Geometry: final body of the model. Coordinates: model frame, mm. A direction names the side the tool comes from. Round coordinates to 2 decimals unless told otherwise and drop trailing zeros. Loops run counter-clockwise (first coordinate to the right, second up) from the corner with the lowest first, then second, coordinate; pieces in that order, holes last. Notation, with made-up numbers: (75, 80) - (83, 80) arc R20 ccw to (83, 94) - close; hole circle Ø8 at (74, 83.25). An arc over 180 degrees is marked (long way). Answer as a JSON object with one key per item and string values. Group by question number.
Item 1: Draft query along X for faces 3 (the face through (32.466, 48.487, -12.836)), 4 (the face through (9.273, 4.93, -17.314)), 5 (the face through (13.25, 48, -13)). Return one class per face: released by +X, released by -X, zero draft, split by the parting line, or undercut.
Item 2: Section C-C (y = 80). Return the cut outline in (x, z), plus the area to 3 significant figures.
Item 3: Section D-D (x = 27). Return the cut outline in (y, z), plus the area to 3 significant figures.
Item 4: Section A-A (y = 67). Return the cut outline in (x, z), plus the area to 4 significant figures.
Item 5: First-contact query: pin 1 (3 mm diameter, centred on y = 70, z = -12.5, fed in from +X); pin 2 (6 mm diameter, centred on x = 5.5, z = -7.5, fed in from +Y); pin 3 (3 mm diameter, centred on y = 27.5, z = -15.5, fed in from -X). Flat tips, straight axial feed; report the tip coordinate or a pass-through.
Item 6: Line query: line 1 (X direction, y = 71, z = -9.5); line 2 (Z direction, x = 19.25, y = 60); line 3 (X direction, y = 15.5, z = -18.5). Output: solid intervals per line, ascending.
Item 7: Reachability of faces 1 (the face through (0, 5, -12)), 2 (the face through (25, 18, -12)) from +Z, -Z, +X, -X, +Y, -Y: full face, straight path, thin tool, end or side. Return the list, or none.
Item 8: Section B-B (z = -7). Return the cut outline in (x, y), plus the area to 3 significant figures.
```python
from build123d import *

# Parameters (mm, degrees)
SKETCH1_W               = 50
SKETCH1_H               = 25
BOSS_EXTRUDE1_DEPTH     = 10
SKETCH2_W               = 20
SKETCH2_H               = 25
BOSS_EXTRUDE2_DEPTH     = 75
SKETCH3_W               = 6.6
SKETCH3_H               = 25
CUT_EXTRUDE1_DEPTH      = 75
SKETCH4_R               = 1.55
CUT_EXTRUDE2_DEPTH      = 96.262794416
LPATTERN1_COUNT         = 6
LPATTERN1_PITCH         = 10
SKETCH5_W               = 15
SKETCH5_H               = 25
CUT_EXTRUDE3_DEPTH      = 94.541434669
SKETCH6_R               = 1.9
CUT_EXTRUDE4_DEPTH      = 96.262794416
SKETCH7_R               = 1.9
CUT_EXTRUDE5_DEPTH      = 87.458082329
SKETCH8_W               = 6.6
SKETCH8_H               = 8
BOSS_EXTRUDE4_DEPTH     = 25
SKETCH11_W              = 25
SKETCH11_H              = 85
BOSS_EXTRUDE5_DEPTH     = 1.75
SKETCH12_W              = 25
SKETCH12_H              = 75
BOSS_EXTRUDE6_DEPTH     = 1.75
SKETCH14_R              = 1.9
CUT_EXTRUDE7_DEPTH      = 88.18120497
CUT_EXTRUDE8_DEPTH      = 94.010160735
CUT_EXTRUDE8_DEPTH_BACK = 94.010160735
SKETCH15_R              = 1.55
CHAMFER1_SIZE           = 1


with BuildPart() as part:
    # Sketch1 → Boss-Extrude1 (new body)
    with BuildSketch(Plane(origin=(0, 0, 0), x_dir=(1, 0, 0), z_dir=(0, 1, 0))):
        with Locations((25, 12.5)):
            Rectangle(SKETCH1_W, SKETCH1_H)
    extrude(amount=BOSS_EXTRUDE1_DEPTH)

    # Sketch2 → Boss-Extrude2 (add)
    with BuildSketch(Plane(origin=(0, 10, 0), x_dir=(1, 0, 0), z_dir=(0, 1, 0))):
        with Locations((25, 12.5)):
            Rectangle(SKETCH2_W, SKETCH2_H)
    extrude(amount=BOSS_EXTRUDE2_DEPTH)

    # Sketch3 → Cut-Extrude1 (cut)
    with BuildSketch(Plane(origin=(0, 85, 0), x_dir=(1, 0, 0), z_dir=(0, 1, 0))):
        with Locations((25, 12.5)):
            Rectangle(SKETCH3_W, SKETCH3_H)
    extrude(amount=-CUT_EXTRUDE1_DEPTH, mode=Mode.SUBTRACT)

    # Sketch4 → Cut-Extrude2 (cut, symmetric)
    with BuildSketch(Plane.ZY.offset(-15)):
        with Locations((-12.5, 80)):
            Circle(SKETCH4_R)
    cut_extrude2 = extrude(amount=CUT_EXTRUDE2_DEPTH, both=True, mode=Mode.SUBTRACT)

    # LPattern1: Cut-Extrude2 ×6
    with Locations(*[(0, -i * LPATTERN1_PITCH, 0) for i in range(1, LPATTERN1_COUNT)]):
        add(cut_extrude2, mode=Mode.SUBTRACT)

    # Sketch5 → Cut-Extrude3 (cut, through all)
    with BuildSketch(Plane(origin=(0, 10, 0), x_dir=(1, 0, 0), z_dir=(0, 1, 0))):
        with Locations((42.5, 12.5)):
            Rectangle(SKETCH5_W, SKETCH5_H)
    extrude(amount=-CUT_EXTRUDE3_DEPTH, mode=Mode.SUBTRACT)

    # Sketch6 → Cut-Extrude4 (cut, through all)
    with BuildSketch(Plane.XZ):
        with Locations(Location((10.000440006, -5.930630913, 0), (0, 0, 270))):
            Circle(SKETCH6_R)
    cut_extrude4 = extrude(amount=-CUT_EXTRUDE4_DEPTH, mode=Mode.SUBTRACT)

    # Mirror1: Cut-Extrude4 across plane
    add(cut_extrude4.mirror(Plane.XY.offset(-12.5)), mode=Mode.SUBTRACT)

    # Sketch7 → Cut-Extrude5 (cut, through all)
    with BuildSketch(Plane(origin=(0, 10, 0), x_dir=(1, 0, 0), z_dir=(0, 1, 0))):
        with Locations(Location((10.000440006, 14.590630913, 0), (0, 0, 270))):
            Circle(SKETCH7_R)
        with Locations(Location((10.000440006, 5.930630913, 0), (0, 0, 90))):
            Circle(SKETCH7_R)
    extrude(amount=-CUT_EXTRUDE5_DEPTH, mode=Mode.SUBTRACT)

    # Sketch8 → Boss-Extrude4 (add, through all)
    with BuildSketch(Plane.XY):
        with Locations((25, 14)):
            Rectangle(SKETCH8_W, SKETCH8_H)
    extrude(amount=-BOSS_EXTRUDE4_DEPTH)

    # Sketch11 → Boss-Extrude5 (add)
    with BuildSketch(Plane(origin=(35, 0, 0), x_dir=(0, 0, -1), z_dir=(1, 0, 0))):
        with Locations((12.5, 42.5)):
            Rectangle(SKETCH11_W, SKETCH11_H)
    extrude(amount=BOSS_EXTRUDE5_DEPTH)

    # Sketch12 → Boss-Extrude6 (add)
    with BuildSketch(Plane.ZY.offset(-15)):
        with Locations((-12.5, 47.5)):
            Rectangle(SKETCH12_W, SKETCH12_H)
    extrude(amount=BOSS_EXTRUDE6_DEPTH)

    # Sketch14 → Cut-Extrude7 (cut, through all)
    with BuildSketch(Plane(origin=(0, 10, 0), x_dir=(1, 0, 0), z_dir=(0, 1, 0))):
        with Locations(Location((10.000440006, 10.260630913, 0), (0, 0, 270))):
            Circle(SKETCH14_R)
    extrude(amount=-CUT_EXTRUDE7_DEPTH, mode=Mode.SUBTRACT)

    # Sketch15 → Cut-Extrude8 (cut, two sides: drawn at the far end of the back side and taken through both)
    with BuildSketch(Plane.ZY.offset(-28.3).offset(-CUT_EXTRUDE8_DEPTH_BACK)):
        with Locations((-12.5, 30)):
            Circle(SKETCH15_R)
        with Locations((-12.5, 40)):
            Circle(SKETCH15_R)
        with Locations((-12.5, 50)):
            Circle(SKETCH15_R)
        with Locations((-12.5, 60)):
            Circle(SKETCH15_R)
        with Locations((-12.5, 70)):
            Circle(SKETCH15_R)
        with Locations((-12.5, 80)):
            Circle(SKETCH15_R)
    extrude(amount=CUT_EXTRUDE8_DEPTH + CUT_EXTRUDE8_DEPTH_BACK, mode=Mode.SUBTRACT)

    # Chamfer1
    chamfer1_edges = [part.edges().sort_by_distance(p)[0] for p in [
        (21.7, 51.5, -25),
        (21.7, 51.5, 0),
        (28.3, 51.5, 0),
        (28.3, 51.5, -25),
        (25, 18, -25),
        (25, 18, 0),
        (36.75, 85, -12.5),
        (36.75, 42.5, 0),
        (36.75, 0, -12.5),
        (36.75, 42.5, -25),
        (6.625, 10, -25),
        (13.25, 47.5, -25),
        (13.25, 47.5, 0),
        (13.25, 85, -12.5),
        (17.475, 85, 0),
        (32.525, 85, -25),
        (32.525, 85, 0),
        (17.475, 85, -25),
        (0, 10, -12.5),
        (18.375, 0, 0),
        (0, 0, -12.5),
        (0, 5, -25),
        (18.375, 0, -25),
        (0, 5, 0),
        (6.625, 10, 0),
    ]]
    chamfer(chamfer1_edges, length=CHAMFER1_SIZE)


solid = part.part
```
Values:
{
 "1": {"face 3": "zero draft", "face 4": "undercut", "face 5": "released by -X"},
 "2": {"outline": "(13.25, -24) - (14.25, -25) - (20.7, -25) - (21.7, -24) - (21.7, -14.05) - (13.25, -14.05) - close; (13.25, -10.95) - (21.7, -10.95) - (21.7, -1) - (20.7, 0) - (14.25, 0) - (13.25, -1) - close; (28.3, -24) - (29.3, -25) - (35.75, -25) - (36.75, -24) - (36.75, -14.05) - (28.3, -14.05) - close; (28.3, -10.95) - (36.75, -10.95) - (36.75, -1) - (35.75, 0) - (29.3, 0) - (28.3, -1) - close", "area": "366 mm^2"},
 "3": {"outline": "(0, -24) - (1, -25) - (17, -25) - (18, -24) - (18, -1) - (17, 0) - (1, 0) - (0, -1) - close", "area": "448 mm^2"},
 "4": {"outline": "(13.25, -24) - (14.25, -25) - (20.7, -25) - (21.7, -24) - (21.7, -1) - (20.7, 0) - (14.25, 0) - (13.25, -1) - close; (28.3, -24) - (29.3, -25) - (35.75, -25) - (36.75, -24) - (36.75, -1) - (35.75, 0) - (29.3, 0) - (28.3, -1) - close", "area": "418.5 mm^2"},
 "5": {"pin 1": "passes through", "pin 2": "stops at y = 10", "pin 3": "stops at x = 13.25"},
 "6": {"line 1": "x = 13.25 to 21.7, 28.3 to 36.75", "line 2": "z = -25 to -14.05, -10.95 to 0", "line 3": "x = 13.25 to 36.75"},
 "7": {"face 1": "+Z, -Z, -X, +Y, -Y", "face 2": "+Z, -Z, +Y"},
 "8": {"outline": "(0, 1) - (1, 0) - (8.43, 0) - (8.43, 10) - (1, 10) - (0, 9) - close; (11.57, 0) - (35.75, 0) - (36.75, 1) - (36.75, 84) - (35.75, 85) - (28.3, 85) - (28.3, 18) - (21.7, 18) - (21.7, 85) - (14.25, 85) - (13.25, 84) - (13.25, 10) - (11.57, 10) - close", "area": "1,650 mm^2"}
}
